from build123d import *

# Parameters (mm, degrees)
SKETCH1_W               = 8
SKETCH1_H               = 15
BOSS_EXTRUDE1_DEPTH     = 3
SKETCH2_R               = 2.5
BOSS_EXTRUDE2_DEPTH     = 7
CUT_EXTRUDE1_DEPTH      = 8
CUT_EXTRUDE1_DEPTH_BACK = 10
SKETCH3_R               = 1.5


with BuildPart() as part:
    # Sketch1 → Boss-Extrude1 (new body)
    with BuildSketch(Plane(origin=(0, 0, 0), x_dir=(1, 0, 0), z_dir=(0, 1, 0))):
        with BuildLine():
            Line((-23, -20), (23, -20))
            ThreePointArc((23, -20), (23.707106781, -19.707106781), (24, -19))
            Line((24, -19), (24, 19))
            ThreePointArc((24, 19), (23.707106781, 19.707106781), (23, 20))
            Line((23, 20), (-23, 20))
            ThreePointArc((-23, 20), (-23.707106781, 19.707106781), (-24, 19))
            Line((-24, 19), (-24, -19))
            ThreePointArc((-24, -19), (-23.707106781, -19.707106781), (-23, -20))
        make_face()
        with Locations((-8, 5.5)):
            Rectangle(SKETCH1_W, SKETCH1_H, mode=Mode.SUBTRACT)
        with Locations((8, 5.5)):
            Rectangle(SKETCH1_W, SKETCH1_H, mode=Mode.SUBTRACT)
    extrude(amount=BOSS_EXTRUDE1_DEPTH)

    # Sketch2 → Boss-Extrude2 (add)
    with BuildSketch(Plane.XZ):
        with Locations(Location((0, -16, 0), (0, 0, 270))):
            Circle(SKETCH2_R)
    extrude(amount=BOSS_EXTRUDE2_DEPTH)

    # Sketch3 → Cut-Extrude1 (cut, two sides: drawn at the far end of the back side and taken through both)
    with BuildSketch(Plane.ZY.offset(-CUT_EXTRUDE1_DEPTH_BACK)):
        with Locations(Location((-16, -4, 0), (0, 0, 180))):
            Circle(SKETCH3_R)
    extrude(amount=CUT_EXTRUDE1_DEPTH + CUT_EXTRUDE1_DEPTH_BACK, mode=Mode.SUBTRACT)


solid = part.part
Geometry check sheet. Reference: the model listing, model coordinates, mm. A direction names the side the tool comes from. Give positions to 0.01 mm unless a question says otherwise; leave off trailing zeros. Write each loop counter-clockwise with the first axis right and the second up, starting at its lowest first coordinate (ties: lowest second). Pieces come first, ordered by that corner, then holes. Notation, with made-up numbers: M 37.5,23.5 L 68.5,23.5 A21 cw 68.5,54.5 Z; hole C 72.5,-25 d5. An arc over 180 degrees is marked long. Answer as CSV lines item,"result". Start each with the question number.
Q1. Go/stop test with flat-tipped pins: pin 1 (3 mm diameter, centred on x = -13.5, y = -1, fed in from +Z); pin 2 (4 mm diameter, centred on x = 16, z = 15.5, fed in from -Y); pin 3 (2.5 mm diameter, centred on y = -4, z = -16, fed in from -X). Record where each tip stops, or that it passes through.
Q2. Material ranges on L1, parallel to X at y = 0.75, z = -10; L2, parallel to Y at x = -0.2, z = -16; L3, parallel to Z at x = -0.1, y = -4, recorded low to high.
Q3. Section check D-D, the plane x = 0. Record the cut outline in (y, z).
Q4. Tool access check on faces 5 (the face through (0.04, -4.07, -14.5)), 6 (the face through (0.1, -3.5, -13.5)), 7 (the face through (8, 1, 2)). Record the directions out of +Z, -Z, +X, -X, +Y, -Y that give a thin tool (end or side, any length) a straight path to the whole face; none if there is none.
Q5. Section check A-A, the plane z = -16. Record the cut outline in (x, y), then the cut area to 3 significant figures.
Q6. Section check B-B, the plane z = -0.5. Record the cut outline in (x, y).
Q7. Section check C-C, the plane y = -4. Record the cut outline in (x, z).
Q8. Release check for a two-part mould opening along Z. For faces 1 (the face through (0, 1, 20)), 2 (the face through (24, 1, 0)), 3 (the face through (-12, 1, -5)), 4 (the face through (0, 1, -20)) record: pulls with the +Z half, pulls with the -Z half, needs draft (parallel to the pull), parting line crosses it, or undercut.
Geometry says:
1,pin 1,"z = 20"
1,pin 2,"y = 0"
1,pin 3,"through"
2,L1,"-24 to -12, -4 to 4, 12 to 24"
2,L2,"-7 to -5.5, -2.5 to 3"
2,L3,"-18.5 to -17.5, -14.5 to -13.5"
3,outline,"M -7,-18.5 L 0,-18.5 L 0,-20 L 3,-20 L 3,20 L 0,20 L 0,-13.5 L -7,-13.5 Z; hole C -4,-16 d3"
4,face 5,"+X, -X"
4,face 6,"-Y"
4,face 7,"+Y, -Y"
5,outline,"M -24,0 L -2.5,0 L -2.5,-2.5 L 2.5,-2.5 L 2.5,0 L 24,0 L 24,3 L -24,3 Z; M -2.5,-7 L 2.5,-7 L 2.5,-5.5 L -2.5,-5.5 Z"
5,area,"164 mm^2"
6,outline,"M -24,0 L -12,0 L -12,3 L -24,3 Z; M -4,0 L 4,0 L 4,3 L -4,3 Z; M 12,0 L 24,0 L 24,3 L 12,3 Z"
7,outline,"M -2,-17.5 A2.5 ccw 2,-17.5 Z; M -2,-14.5 L 2,-14.5 A2.5 ccw Z"
8,face 1,"pulls with the +Z half"
8,face 2,"needs draft"
8,face 3,"undercut"
8,face 4,"pulls with the -Z half"
